```python
from build123d import *

# Parameters (mm, degrees)
CROQUIS1_R              = 1.5
SALIENTE_EXTRUIR1_DEPTH = 3
CROQUIS3_W              = 22
CROQUIS3_H              = 37
SALIENTE_EXTRUIR2_DEPTH = 13
CORTAR_EXTRUIR1_START   = -37
CORTAR_EXTRUIR1_DEPTH   = 37
SALIENTE_EXTRUIR4_DEPTH = 6
CROQUIS7_W              = 3.002058729
CROQUIS7_H              = 21
CORTAR_EXTRUIR2_DEPTH   = 22
CROQUIS8_W              = 3
CROQUIS8_H              = 43
SALIENTE_EXTRUIR5_DEPTH = 25
SALIENTE_EXTRUIR6_START = -19
SALIENTE_EXTRUIR6_DEPTH = 19
CROQUIS13_W             = 1
CROQUIS13_H             = 2
CROQUIS13_H_2           = 5
SALIENTE_EXTRUIR8_DEPTH = 1.5


with BuildPart() as part:
    # Croquis1 → Saliente-Extruir1 (new body)
    with BuildSketch(Plane.XY):
        with BuildLine():
            Line((-4.197309417, 33.461883408), (-52.197309417, 33.461883408))
            ThreePointArc((-52.197309417, 33.461883408), (-55.025736542, 32.290310533), (-56.197309417, 29.461883408))
            Line((-56.197309417, 29.461883408), (-56.197309417, 24.961883408))
            Line((-56.197309417, 24.961883408), (-49.197309417, 24.961883408))
            Line((-49.197309417, 24.961883408), (-49.197309417, 4.961883408))
            Line((-49.197309417, 4.961883408), (-56.197309417, 4.961883408))
            Line((-56.197309417, 4.961883408), (-56.197309417, 0.461883408))
            ThreePointArc((-56.197309417, 0.461883408), (-55.099110766, -2.293519818), (-52.406664651, -3.538116592))
            Line((-52.406664651, -3.538116592), (-4.197309417, -3.538116592))
            Line((-4.197309417, -3.538116592), (-4.197309417, 7.961883408))
            Line((-4.197309417, 7.961883408), (-10.197309417, 7.961883408))
            Line((-10.197309417, 7.961883408), (-10.197309417, 21.961883408))
            Line((-10.197309417, 21.961883408), (-4.197309417, 21.961883408))
            Line((-4.197309417, 21.961883408), (-4.197309417, 33.461883408))
        make_face()
        with Locations((-52.19152813, 0.461883408)):
            Circle(CROQUIS1_R, mode=Mode.SUBTRACT)
        with Locations((-7.69152813, 0.461883408)):
            Circle(CROQUIS1_R, mode=Mode.SUBTRACT)
        with Locations((-52.197309417, 29.461883408)):
            Circle(CROQUIS1_R, mode=Mode.SUBTRACT)
        with Locations((-7.697309417, 29.461882832)):
            Circle(CROQUIS1_R, mode=Mode.SUBTRACT)
    extrude(amount=SALIENTE_EXTRUIR1_DEPTH)

    # Croquis3 → Saliente-Extruir2 (add)
    with BuildSketch(Plane.XY.offset(3)):
        with Locations((-38.197309417, 14.961883408)):
            Rectangle(CROQUIS3_W, CROQUIS3_H)
    extrude(amount=SALIENTE_EXTRUIR2_DEPTH)

    # Croquis4 → Cortar-Extruir1 (cut)
    with BuildSketch(Plane.XZ.offset(3.538116592).offset(CORTAR_EXTRUIR1_START)):
        Polygon((-27.197309417, 16), (-27.197309417, 6.002058729), (-49.197309417, 16), align=None)
    extrude(amount=CORTAR_EXTRUIR1_DEPTH, mode=Mode.SUBTRACT)

    # Croquis6 → Saliente-Extruir4 (add)
    with BuildSketch(Plane(origin=(0, 33.461883408, 0), x_dir=(1, 0, 0), z_dir=(0, 1, 0))):
        Polygon((-27.197309417, -6.002058729), (-49.197309417, -16), (-49.197309417, 0), (-27.197309417, 0), align=None)
    extrude(amount=SALIENTE_EXTRUIR4_DEPTH)

    # Croquis7 → Cortar-Extruir2 (cut)
    with BuildSketch(Plane(origin=(-27.197309417, 0, 0), x_dir=(0, 0, -1), z_dir=(1, 0, 0))):
        with Locations((-4.501029365, 25.961883408)):
            Rectangle(CROQUIS7_W, CROQUIS7_H)
    extrude(amount=-CORTAR_EXTRUIR2_DEPTH, mode=Mode.SUBTRACT)

    # Croquis8 → Saliente-Extruir5 (add)
    with BuildSketch(Plane(origin=(-2.394740987, 0, -5.269515022), x_dir=(0.9103985682863143, 0, -0.4137323372208525), z_dir=(0.4137323372208525, 0, 0.9103985682863143))):
        with Locations((-28.743637341, 17.961883408)):
            Rectangle(CROQUIS8_W, CROQUIS8_H)
    extrude(amount=SALIENTE_EXTRUIR5_DEPTH)

    # Croquis9 → Saliente-Extruir6 (add)
    with BuildSketch(Plane.XZ.offset(3.538116592).offset(SALIENTE_EXTRUIR6_START)):
        Polygon((-16.854000987, 28.762022936), (-27.197309417, 6.002058729), (-27.197309417, 3), (-16.854000987, 3), align=None)
    extrude(amount=SALIENTE_EXTRUIR6_DEPTH)

    # Croquis13 → Saliente-Extruir8 (add)
    with BuildSketch(Plane.XY.offset(3)):
        with Locations((-10.197309417, -2.538116592)):
            Rectangle(CROQUIS13_W, CROQUIS13_H)
        with Locations((-10.197309417, 32.461883408)):
            Rectangle(CROQUIS13_W, CROQUIS13_H)
        with Locations((-14.197309417, 30.961883408)):
            Rectangle(CROQUIS13_W, CROQUIS13_H_2)
        with Locations((-14.197309417, -1.038116592)):
            Rectangle(CROQUIS13_W, CROQUIS13_H_2)
    extrude(amount=SALIENTE_EXTRUIR8_DEPTH)


solid = part.part
```
The listing builds one solid part. Answer for the finished solid, in the listing's coordinates (mm). A direction names the side the tool comes from. Give positions to 0.01 mm unless a question says otherwise; leave off trailing zeros. Loops run counter-clockwise (first coordinate to the right, second up) from the corner with the lowest first, then second, coordinate; pieces in that order, holes last. Notation, with made-up numbers: (-31, -1.75) - (10, -1.75) arc R11 cw to (10, 6.25) - close; hole circle Ø5 at (71.5, 88.25). An arc over 180 degrees is marked (long way). Answer as CSV lines item,"result". Start each with the question number.
Item 1: For faces 5 (the face through (-14.697, 31, 4)), 6 (the face through (-30, 21, 3)), 7 (the face through (-10.197, 15, 1)), 8 (the face through (-9.697, 32, 4)), 9 (the face through (-53, 4.962, 1)), determine the directions among +Z, -Z, +X, -X, +Y, -Y from which every point of the face is accessible in a straight line to the end or side of a thin tool.
Item 2: A cutting plane is placed at A-A on y = 35. Determine the outline of the cut face in (x, z), then the cut area to 3 significant figures.
Item 3: Each of these flat-tipped pins is pushed along its axis until it touches: pin 1 (9.5 mm diameter, centred on y = 8, z = 16.5, fed in from +X); pin 2 (12 mm diameter, centred on x = -20, y = 22.5, fed in from +Z); pin 3 (0.8 mm diameter, centred on y = 32, z = 4, fed in from -X). Where does it stop, or does it pass through?
Item 4: A cutting plane is placed at D-D on x = -44.5. Determine the outline of the cut face in (y, z).
Item 5: A cutting plane is placed at C-C on y = 7. Determine the outline of the cut face in (x, z).
Item 6: The mould has two halves that part along X. Classify faces 1 (the face through (-13.697, 31, 4)), 2 (the face through (-18.24, 18.26, 29.39)), 3 (the face through (-39.43, 17.66, 11.56)), 4 (the face through (-28.6, -3.538, 8.5)): +X half, -X half, draft (parallel to the pull), parting line (faces both ways), or undercut.
Item 7: Find the intervals of material crossed by line 1 (Y direction, x = -38, z = 5); line 2 (Z direction, x = -27, y = 25.5); line 3 (Z direction, x = -20, y = 28.5), in increasing order. Write a range as from..to.
Item 8: A cutting plane is placed at B-B on z = 12. Determine the outline of the cut face in (x, y), then the cut area to 3 significant figures.
Found:
1,face 5,"+Z, -X, +Y, -Y"
1,face 6,"none"
1,face 7,"+Z, -Z, +X"
1,face 8,"+Z, +X, +Y, -Y"
1,face 9,"+Z, -Z, -X"
2,outline,"(-49.2, 0) - (-27.2, 0) - (-27.2, 3) - (-49.2, 3) - close; (-49.2, 6) - (-27.2, 6) - (-16.85, 28.76) - (-19.59, 30) - (-29.93, 7.24) - (-49.2, 16) - close"
2,area,"251 mm^2"
3,pin 1,"stops at x = -16.85"
3,pin 2,"stops at z = 30"
3,pin 3,"stops at x = -14.7"
4,outline,"(-3.54, 0) - (39.46, 0) - (39.46, 13.87) - (-3.54, 13.87) - close; hole (15.46, 3) - (36.46, 3) - (36.46, 6) - (15.46, 6) - close"
5,outline,"(-49.2, 0) - (-4.2, 0) - (-4.2, 3) - (-16.85, 3) - (-16.85, 28.76) - (-19.59, 30) - (-29.93, 7.24) - (-49.2, 16) - close"
6,face 1,"undercut"
6,face 2,"+X half"
6,face 3,"undercut"
6,face 4,"draft"
7,line 1,"y = -3.54..15.46, 36.46..39.46"
7,line 2,"z = 0..3, 6.44..13.69"
7,line 3,"z = 0..3, 21.84..29.09"
8,outline,"(-49.2, -3.54) - (-40.4, -3.54) - (-40.4, 39.46) - (-49.2, 39.46) - close; (-27.77, -3.54) - (-16.85, -3.54) - (-16.85, 15.46) - (-24.47, 15.46) - (-24.47, 39.46) - (-27.77, 39.46) - close"
8,area,"665 mm^2"
